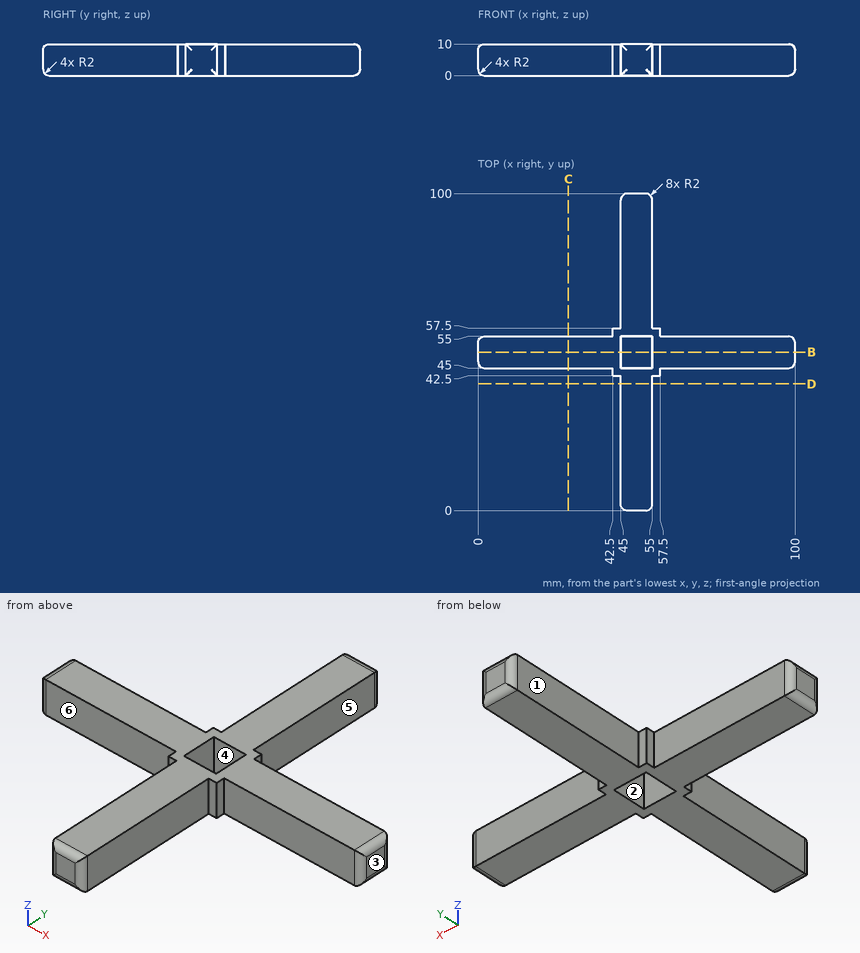
Input: dimensioned drawing with shaded views. Units: mm. Origin: part minimum x, y, z. A direction names the side the tool comes from. Round coordinates to 2 decimals unless told otherwise and drop trailing zeros. Order: outer loops, then holes, each group sorted by start corner. A loop starts at its lowest first (then second) coordinate and runs counter-clockwise, first axis right, second up.
Q1. Pin query (flat end, axial travel): pin 1 (12 mm diameter, centred on x = 38.5, y = 39.5, fed in from -Z); pin 2 (0.8 mm diameter, centred on y = 55.5, z = 5.5, fed in from -X); pin 3 (0.8 mm diameter, centred on x = 56.5, z = 4.5, fed in from -Y); pin 4 (3 mm diameter, centred on y = 74.5, z = 4.5, fed in from +X). Return the tip coordinate at first contact, or that it passes through.
Result sheet:
pin 1: stops at z = 0
pin 2: stops at x = 42.5
pin 3: stops at y = 42.5
pin 4: stops at x = 55
Q2. Access query for the marked faces 4, 5 and 6. Directions: +Z, -Z, +X, -X, +Y, -Y. A direction counts if a zero-diameter tool reaches every point of the face in a straight line with its end or side. Return the directions, or none.
Result sheet:
face 4: +Z, -Z
face 5: +Z, -Z, +X, +Y
face 6: +Z, -Z, -X, -Y
Q3. Section B-B, the plane y = 50. Output: boundary loops of the cut face in (x, z), and give its area (3 significant figures).
Result sheet:
outline: (0, 2) arc R2 ccw to (2, 0) - (45, 0) - (45, 10) - (2, 10) arc R2 ccw to (0, 8) - close; (55, 0) - (98, 0) arc R2 ccw to (100, 2) - (100, 8) arc R2 ccw to (98, 10) - (55, 10) - close
area: 897 mm2
Q4. Material intervals for probe 1 along X at (y, z) = (49.5, 3.5); probe 2 along Y at (x, z) = (35, 3.75), sorted ascending.
Result sheet:
probe 1: x = 0 to 45, 55 to 100
probe 2: y = 45 to 55
Q5. Mould query, pull axis X, two halves, no side actions, for the marked faces 1, 2 and 3. Classes: released by +X, released by -X, zero draft, split by the parting line, or undercut.
Result sheet:
face 1: released by -X
face 2: undercut
face 3: released by +X
Q6. Section C-C, the plane x = 28.5. Output: boundary loops of the cut face in (y, z), and give its area (3 significant figures).
Result sheet:
outline: (45, 0) - (55, 0) - (55, 10) - (45, 10) - close
area: 100 mm2
